```python
from build123d import *

# Parameters (mm, degrees)
SKETCH1_W               = 77.6
SKETCH1_H               = 61.3
BOSS_EXTRUDE1_DEPTH     = 7
SKETCH2_W               = 95.2
SKETCH2_H               = 78.9
SKETCH2_W_2             = 75.2
SKETCH2_H_2             = 58.9
CUT_EXTRUDE_THIN1_DEPTH = 1.85
SKETCH3_W               = 73.6
SKETCH3_H               = 57.3
CUT_EXTRUDE1_DEPTH      = 5
SKETCH4_W               = 13.5
SKETCH4_H               = 2.85
SKETCH4_W_2             = 10.5
CUT_EXTRUDE2_DEPTH      = 5
FILLET1_R               = 1
CUT_EXTRUDE3_REACH      = 51.698
SKETCH5_W               = 20.41
SKETCH5_H               = 2.7
SKETCH5_W_2             = 15.3
SKETCH5_W_3             = 20.5
SKETCH5_W_4             = 25.49
SKETCH6_R               = 2.5
BOSS_EXTRUDE2_DEPTH     = 13.5
SKETCH7_R               = 1
CUT_EXTRUDE4_DEPTH      = 5
CUT_EXTRUDE5_REACH      = 53.255
SKETCH8_R               = 1


with BuildPart() as part:
    # Sketch1 → Boss-Extrude1 (new body)
    with BuildSketch(Plane(origin=(0, 0, 0), x_dir=(1, 0, 0), z_dir=(0, 1, 0))):
        Rectangle(SKETCH1_W, SKETCH1_H)
    extrude(amount=BOSS_EXTRUDE1_DEPTH)

    # Sketch2 → Cut-Extrude-Thin1 (cut)
    with BuildSketch(Plane(origin=(0, 7, 0), x_dir=(1, 0, 0), z_dir=(0, 1, 0))):
        Rectangle(SKETCH2_W, SKETCH2_H)
        Rectangle(SKETCH2_W_2, SKETCH2_H_2, mode=Mode.SUBTRACT)
    extrude(amount=-CUT_EXTRUDE_THIN1_DEPTH, mode=Mode.SUBTRACT)

    # Sketch3 → Cut-Extrude1 (cut)
    with BuildSketch(Plane(origin=(0, 7, 0), x_dir=(1, 0, 0), z_dir=(0, 1, 0))):
        Rectangle(SKETCH3_W, SKETCH3_H)
    extrude(amount=-CUT_EXTRUDE1_DEPTH, mode=Mode.SUBTRACT)

    # Sketch4 → Cut-Extrude2 (cut)
    with BuildSketch(Plane.ZY.offset(38.8)):
        with Locations((11.45, 5.575)):
            Rectangle(SKETCH4_W, SKETCH4_H)
        with Locations((-18.4, 5.575)):
            Rectangle(SKETCH4_W_2, SKETCH4_H)
    extrude(amount=-CUT_EXTRUDE2_DEPTH, mode=Mode.SUBTRACT)

    # Fillet1
    fillet1_edges = [part.edges().sort_by_distance(p)[0] for p in [
        (38.8, 2.575, 30.65),
        (-38.8, 2.575, 30.65),
        (-38.8, 2.575, -30.65),
        (38.8, 2.575, -30.65),
        (36.8, 2, 0),
        (36.8, 4.5, -28.65),
        (0, 2, 28.65),
        (36.8, 4.5, 28.65),
        (-36.8, 2, 0),
        (-36.8, 4.5, 28.65),
        (0, 2, -28.65),
        (-36.8, 4.5, -28.65),
        (0, 0, 30.65),
        (-38.8, 0, 0),
        (0, 0, -30.65),
        (38.8, 0, 0),
    ]]
    fillet(fillet1_edges, radius=FILLET1_R)

    # Sketch5 → Cut-Extrude3 (cut, up to next)
    with BuildSketch(Plane(origin=(0, 2, 0), x_dir=(1, 0, 0), z_dir=(0, 1, 0)), mode=Mode.PRIVATE) as cut_extrude3_sk1:
        with Locations((20.095, -24.3)):
            Rectangle(SKETCH5_W, SKETCH5_H)
    cut_extrude3_tool1 = extrude(cut_extrude3_sk1.sketch, amount=-CUT_EXTRUDE3_REACH, mode=Mode.PRIVATE) & part.part
    # Sketch5 → Cut-Extrude3 (cut, up to next)
    with BuildSketch(Plane(origin=(0, 2, 0), x_dir=(1, 0, 0), z_dir=(0, 1, 0)), mode=Mode.PRIVATE) as cut_extrude3_sk2:
        with Locations((22.65, 24.6)):
            Rectangle(SKETCH5_W_2, SKETCH5_H)
    cut_extrude3_tool2 = extrude(cut_extrude3_sk2.sketch, amount=-CUT_EXTRUDE3_REACH, mode=Mode.PRIVATE) & part.part
    # Sketch5 → Cut-Extrude3 (cut, up to next)
    with BuildSketch(Plane(origin=(0, 2, 0), x_dir=(1, 0, 0), z_dir=(0, 1, 0)), mode=Mode.PRIVATE) as cut_extrude3_sk3:
        with Locations((2.25, 24.6)):
            Rectangle(SKETCH5_W_3, SKETCH5_H)
    cut_extrude3_tool3 = extrude(cut_extrude3_sk3.sketch, amount=-CUT_EXTRUDE3_REACH, mode=Mode.PRIVATE) & part.part
    # Sketch5 → Cut-Extrude3 (cut, up to next)
    with BuildSketch(Plane(origin=(0, 2, 0), x_dir=(1, 0, 0), z_dir=(0, 1, 0)), mode=Mode.PRIVATE) as cut_extrude3_sk4:
        with Locations((-4.355, -24.3)):
            Rectangle(SKETCH5_W_4, SKETCH5_H)
    cut_extrude3_tool4 = extrude(cut_extrude3_sk4.sketch, amount=-CUT_EXTRUDE3_REACH, mode=Mode.PRIVATE) & part.part
    add(cut_extrude3_tool1.solids().sort_by_distance((20.095, 2, 24.3))[0], mode=Mode.SUBTRACT)
    add(cut_extrude3_tool2.solids().sort_by_distance((22.65, 2, -24.6))[0], mode=Mode.SUBTRACT)
    add(cut_extrude3_tool3.solids().sort_by_distance((2.25, 2, -24.6))[0], mode=Mode.SUBTRACT)
    add(cut_extrude3_tool4.solids().sort_by_distance((-4.355, 2, 24.3))[0], mode=Mode.SUBTRACT)

    # Sketch6 → Boss-Extrude2 (add)
    with BuildSketch(Plane(origin=(0, 2, 0), x_dir=(1, 0, 0), z_dir=(0, 1, 0))):
        with Locations(Location((31.6, 19.09, 0), (0, 0, 270))):
            Circle(SKETCH6_R)
        with Locations(Location((31.6, -8.85, 0), (0, 0, 270))):
            Circle(SKETCH6_R)
        with Locations(Location((-19.5, -24.01, 0), (0, 0, 16.260204708))):
            Circle(SKETCH6_R)
        with Locations(Location((-20.8, 24.19, 0), (0, 0, 270))):
            Circle(SKETCH6_R)
    extrude(amount=BOSS_EXTRUDE2_DEPTH)

    # Sketch7 → Cut-Extrude4 (cut)
    with BuildSketch(Plane(origin=(0, 15.5, 0), x_dir=(1, 0, 0), z_dir=(0, 1, 0))):
        with Locations(Location((31.6, 19.09, 0), (0, 0, 270))):
            Circle(SKETCH7_R)
        with Locations(Location((31.6, -8.85, 0), (0, 0, 270))):
            Circle(SKETCH7_R)
        with Locations(Location((-20.8, 24.19, 0), (0, 0, 270))):
            Circle(SKETCH7_R)
        with Locations(Location((-19.5, -24.01, 0), (0, 0, 270))):
            Circle(SKETCH7_R)
    extrude(amount=-CUT_EXTRUDE4_DEPTH, mode=Mode.SUBTRACT)

    # Sketch8 → Cut-Extrude5 (cut, up to next)
    with BuildSketch(Plane(origin=(0, 2, 0), x_dir=(1, 0, 0), z_dir=(0, 1, 0)), mode=Mode.PRIVATE) as cut_extrude5_sk1:
        with Locations(Location((-28.5, -22.95, 0), (0, 0, 270))):
            Circle(SKETCH8_R)
    cut_extrude5_tool1 = extrude(cut_extrude5_sk1.sketch, amount=-CUT_EXTRUDE5_REACH, mode=Mode.PRIVATE) & part.part
    add(cut_extrude5_tool1.solids().sort_by_distance((-28.5, 2, 22.95))[0], mode=Mode.SUBTRACT)


solid = part.part
```
Input: part model. Units: mm. Frame: model coordinates. A direction names the side the tool comes from. Give positions to 0.01 mm unless a question says otherwise; leave off trailing zeros. Order: outer loops, then holes, each group sorted by start corner. A loop starts at its lowest first (then second) coordinate and runs counter-clockwise, first axis right, second up. Notation, with made-up numbers: M -13,83 L -8,83 A32 ccw -8,113 Z; hole C 76.25,5.25 d4. An arc over 180 degrees is marked long. Return JSON: item names as keys, results as strings.
1) Line query: L1, parallel to X at y = 3.5, z = 0.5; L2, parallel to X at y = 14.5, z = 8.85; L3, parallel to Y at x = 24, z = 14. Output: solid intervals per line, ascending. Write a range as [from, to].
Taken from the geometry:
{"L1": "x = [-38.8, -36.8], [36.8, 38.8]", "L2": "x = [29.1, 30.6], [32.6, 34.1]", "L3": "y = [0, 2]"}
2) Section query C-C on x = -14. Output: boundary loops of the cut face in (y, z).
Taken from the geometry:
{"outline": "M 0,-29.65 A1 ccw 1,-30.65 L 5.15,-30.65 L 5.15,-29.45 L 7,-29.45 L 7,-28.65 L 3,-28.65 A1 cw 2,-27.65 L 2,22.95 L 0,22.95 Z; M 0,25.65 L 2,25.65 L 2,27.65 A1 cw 3,28.65 L 7,28.65 L 7,29.45 L 5.15,29.45 L 5.15,30.65 L 1,30.65 A1 ccw 0,29.65 Z"}
3) Section query D-D on z = -19.09. Output: boundary loops of the cut face in (x, y).
Taken from the geometry:
{"outline": "M -38.8,1 A1 ccw -37.8,0 L 37.8,0 A1 ccw 38.8,1 L 38.8,5.15 L 37.6,5.15 L 37.6,7 L 36.8,7 L 36.8,3 A1 cw 35.8,2 L 34.1,2 L 34.1,15.5 L 32.6,15.5 L 32.6,10.5 L 30.6,10.5 L 30.6,15.5 L 29.1,15.5 L 29.1,2 L -35.8,2 A1 cw -36.8,3 L -36.8,4.15 L -38.8,4.15 Z"}
4) Access query for faces 1 (the face through (-37.6, 6, -4)), 2 (the face through (-38, 5, 18.2)), 3 (the face through (-17.1, 1, 24)), 4 (the face through (-1, 5, -28.65)), 5 (the face through (23, 1, -25.95)). Directions: +Z, -Z, +X, -X, +Y, -Y. A direction counts if a zero-diameter tool reaches every point of the face in a straight line with its end or side. Return the directions, or none.
Taken from the geometry:
{"face 1": "+Z, -Z, -X, +Y", "face 2": "-X, +Y", "face 3": "-Y", "face 4": "+Y", "face 5": "+Y, -Y"}
5) Section query A-A on y = 12.75. Output: boundary loops of the cut face in (x, z).
Taken from the geometry:
{"outline": "C -20.8,-24.19 d5; C -19.5,24.01 d5; C 31.6,-19.09 d5; C 31.6,8.85 d5; hole C -20.8,-24.19 d2; hole C -19.5,24.01 d2; hole C 31.6,-19.09 d2; hole C 31.6,8.85 d2"}
6) Mould query, pull axis Z, two halves, no side actions, for faces 6 (the face through (-38, 5, -23.65)), 7 (the face through (-1, 6, 29.45)), 8 (the face through (-1, 6, -29.45)), 9 (the face through (-38, 4.15, -18)). Classes: released by +Z, released by -Z, zero draft, split by the parting line, or undercut.
Taken from the geometry:
{"face 6": "undercut", "face 7": "released by +Z", "face 8": "released by -Z", "face 9": "undercut"}
7) Contact query for flat-ended pins moving along their axis: pin 1 (10 mm diameter, centred on x = 4, z = 11.5, fed in from +Y); pin 2 (1.8 mm diameter, centred on x = -20.8, z = -24.19, fed in from -Y); pin 3 (0.6 mm diameter, centred on y = 6.5, z = -4.5, fed in from -X); pin 4 (1 mm diameter, centred on x = -37.5, z = 13, fed in from +Y). Output: stop coordinate, or through.
Taken from the geometry:
{"pin 1": "stops at y = 2", "pin 2": "stops at y = 0", "pin 3": "stops at x = -37.6", "pin 4": "stops at y = 4.15"}
8) Section query B-B on x = 7. Output: boundary loops of the cut face in (y, z), and give its area (3 significant figures).
Taken from the geometry:
{"outline": "M 0,-29.65 A1 ccw 1,-30.65 L 5.15,-30.65 L 5.15,-29.45 L 7,-29.45 L 7,-28.65 L 3,-28.65 A1 cw 2,-27.65 L 2,-25.95 L 0,-25.95 Z; M 0,-23.25 L 2,-23.25 L 2,22.95 L 0,22.95 Z; M 0,25.65 L 2,25.65 L 2,27.65 A1 cw 3,28.65 L 7,28.65 L 7,29.45 L 5.15,29.45 L 5.15,30.65 L 1,30.65 A1 ccw 0,29.65 Z", "area": "127 mm2"}
